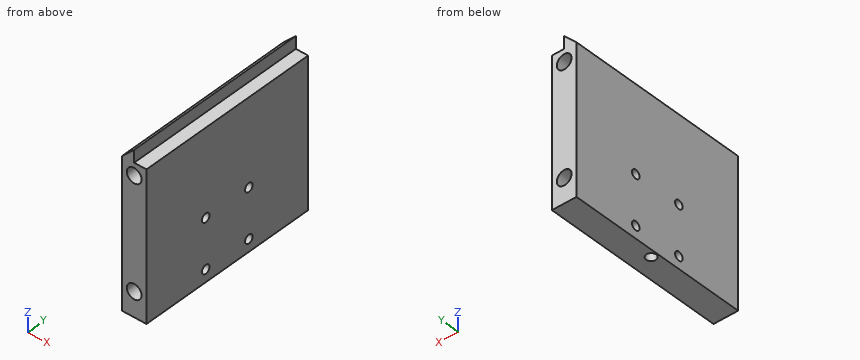
from build123d import *

# Parameters (mm, degrees)
F1_DEPTH  = 75
F3_R      = 1.75
F4_DEPTH  = 25
F6_R      = 3
F7_DEPTH  = 20
F8_R      = 3
F9_DEPTH  = 20
F10_R     = 3
F11_DEPTH = 20
F12_R     = 3
F13_DEPTH = 20
F2_R      = 2
F14_DEPTH = 10
F15_DEPTH = 25
F16_DEPTH = 25
F17_DEPTH = 25


with BuildPart() as f1:
    # F0 (on Front) → F1 (new body)
    with BuildSketch(Plane.XZ):
        Polygon((-5, 27.5), (-5, -32.5), (5, -32.5), (5, 27.5), (0, 27.5), (0, 32.5), align=None)
    extrude(amount=F1_DEPTH)

    # F3 (on face) → F4 (cut)
    with BuildSketch(Plane.YZ.offset(5)):
        with Locations((-27.5, -7.5)):
            Circle(F3_R)
        with Locations((-47.5, -7.5)):
            Circle(F3_R)
        with Locations((-27.5, -27.5)):
            Circle(F3_R)
        with Locations((-47.5, -27.5)):
            Circle(F3_R)
    extrude(amount=-F4_DEPTH, mode=Mode.SUBTRACT)

    # F6 (on face) → F7 (cut)
    with BuildSketch(Plane(origin=(0, 0, 0), x_dir=(-1, 0, 0), z_dir=(0, 1, 0))):
        with Locations((0, -22.5)):
            Circle(F6_R)
    extrude(amount=-F7_DEPTH, mode=Mode.SUBTRACT)

    # F8 (on face) → F9 (cut)
    with BuildSketch(Plane.XZ.offset(75)):
        with Locations((0, 22.5)):
            Circle(F8_R)
    extrude(amount=-F9_DEPTH, mode=Mode.SUBTRACT)

    # F10 (on face) → F11 (cut)
    with BuildSketch(Plane.XZ.offset(75)):
        with Locations((0, -22.5)):
            Circle(F10_R)
    extrude(amount=-F11_DEPTH, mode=Mode.SUBTRACT)

    # F12 (on face) → F13 (cut)
    with BuildSketch(Plane(origin=(0, 0, 0), x_dir=(-1, 0, 0), z_dir=(0, 1, 0))):
        with Locations((0, 22.5)):
            Circle(F12_R)
    extrude(amount=-F13_DEPTH, mode=Mode.SUBTRACT)

    # F2 (on face) → F14 (cut)
    with BuildSketch(Plane(origin=(0, 0, -32.5), x_dir=(1, 0, 0), z_dir=(0, 0, -1))):
        with Locations((-2.5, 37.5)):
            Circle(F2_R)
    extrude(amount=-F14_DEPTH, mode=Mode.SUBTRACT)

    # F3 (on face) → F15 (cut)
    with BuildSketch(Plane.YZ.offset(5)):
        with Locations((-27.5, -7.5)):
            Circle(F3_R)
        with Locations((-47.5, -7.5)):
            Circle(F3_R)
        with Locations((-27.5, -27.5)):
            Circle(F3_R)
        with Locations((-47.5, -27.5)):
            Circle(F3_R)
    extrude(amount=-F15_DEPTH, mode=Mode.SUBTRACT)

    # F3 (on face) → F16 (cut)
    with BuildSketch(Plane.YZ.offset(5)):
        with Locations((-27.5, -7.5)):
            Circle(F3_R)
        with Locations((-47.5, -7.5)):
            Circle(F3_R)
        with Locations((-27.5, -27.5)):
            Circle(F3_R)
        with Locations((-47.5, -27.5)):
            Circle(F3_R)
    extrude(amount=-F16_DEPTH, mode=Mode.SUBTRACT)

    # F3 (on face) → F17 (cut)
    with BuildSketch(Plane.YZ.offset(5)):
        with Locations((-27.5, -7.5)):
            Circle(F3_R)
        with Locations((-47.5, -7.5)):
            Circle(F3_R)
        with Locations((-27.5, -27.5)):
            Circle(F3_R)
        with Locations((-47.5, -27.5)):
            Circle(F3_R)
    extrude(amount=-F17_DEPTH, mode=Mode.SUBTRACT)


solid = f1.part
Can you work these out from the model? Positions are in its coordinate system, mm. Give positions to 0.01 mm unless a question says otherwise; leave off trailing zeros. Loops run counter-clockwise (first coordinate to the right, second up) from the corner with the lowest first, then second, coordinate; pieces in that order, holes last. Notation, with made-up numbers: (14.5, 30.25) -> (33.5, 30.25) arc R22 ccw to (33.5, 66.25) -> close; hole circle Ø10 at (16, 79). An arc over 180 degrees is marked (long way). Write item = value, one per line.
1) Will these pins go through, and if not, where does the flat tip stop? pin 1 (2.5 mm diameter, centred on x = -2.5, y = -37.5, fed in from +Z); pin 2 (3 mm diameter, centred on x = 0, z = -22.5, fed in from +Y); pin 3 (3.5 mm diameter, centred on x = 0, z = -22.5, fed in from -Y).
Check result:
pin_1 = 31.25
pin_2 = -20
pin_3 = -55
2) Suppose I cut it at B-B on y = -27.5. Write out the boundary of the cut face in (x, z).
Check result:
outline = (-5, -32.5) -> (5, -32.5) -> (5, -29.25) -> (-5, -29.25) -> close; (-5, -25.75) -> (5, -25.75) -> (5, -9.25) -> (-5, -9.25) -> close; (-5, -5.75) -> (5, -5.75) -> (5, 27.5) -> (0, 27.5) -> (0, 32.5) -> (-5, 27.5) -> close
3) Suppose I cut it at D-D on y = -37.5. Write out the boundary of the cut face in (x, z).
Check result:
outline = (-5, -32.5) -> (-4.5, -32.5) -> (-4.5, -22.5) -> (-0.5, -22.5) -> (-0.5, -32.5) -> (5, -32.5) -> (5, 27.5) -> (0, 27.5) -> (0, 32.5) -> (-5, 27.5) -> close
4) Suppose I cut it at C-C on y = -11. Write out the boundary of the cut face in (x, z).
Check result:
outline = (-5, -32.5) -> (5, -32.5) -> (5, 27.5) -> (0, 27.5) -> (0, 32.5) -> (-5, 27.5) -> close; hole circle Ø6 at (0, -22.5); hole circle Ø6 at (0, 22.5)
5) I need wall thicknesses on L1, parallel to Z at x = -0.5, y = -13.5; L2, parallel to Z at x = -2.5, y = -47; L3, parallel to Z at x = 2.25, y = -23. Which ranges of each line are inside material? Lowest first, please. Write a range as from..to.
Check result:
L1 = -32.5..-25.46, -19.54..19.54, 25.46..32
L2 = -32.5..-29.18, -25.82..-9.18, -5.82..30
L3 = -32.5..27.5
6) Suppose I cut it at A-A on z = -27.5. Write out the boundary of the cut face in (x, y), then the cut area to 3 significant figures.
Check result:
outline = (-5, -75) -> (5, -75) -> (5, -49.25) -> (-5, -49.25) -> close; (-5, -45.75) -> (5, -45.75) -> (5, -29.25) -> (-5, -29.25) -> close; (-5, -25.75) -> (5, -25.75) -> (5, 0) -> (-5, 0) -> close; hole circle Ø4 at (-2.5, -37.5)
area = 667 mm2
